Part print with two shaded views. Sizes in mm from the minimum x, y, z corner. A direction names the side the tool comes from. Coordinates: 2 decimals unless noted, no trailing zeros. Loops run counter-clockwise (first coordinate to the right, second up) from the corner with the lowest first, then second, coordinate; pieces in that order, holes last. Notation, with made-up numbers: (-11, 0) -> (15, 0) arc R26 cw to (15, 15) -> close; hole circle Ø10 at (55.5, 38). An arc over 180 degrees is marked (long way). Use one line per item in the form item = value.
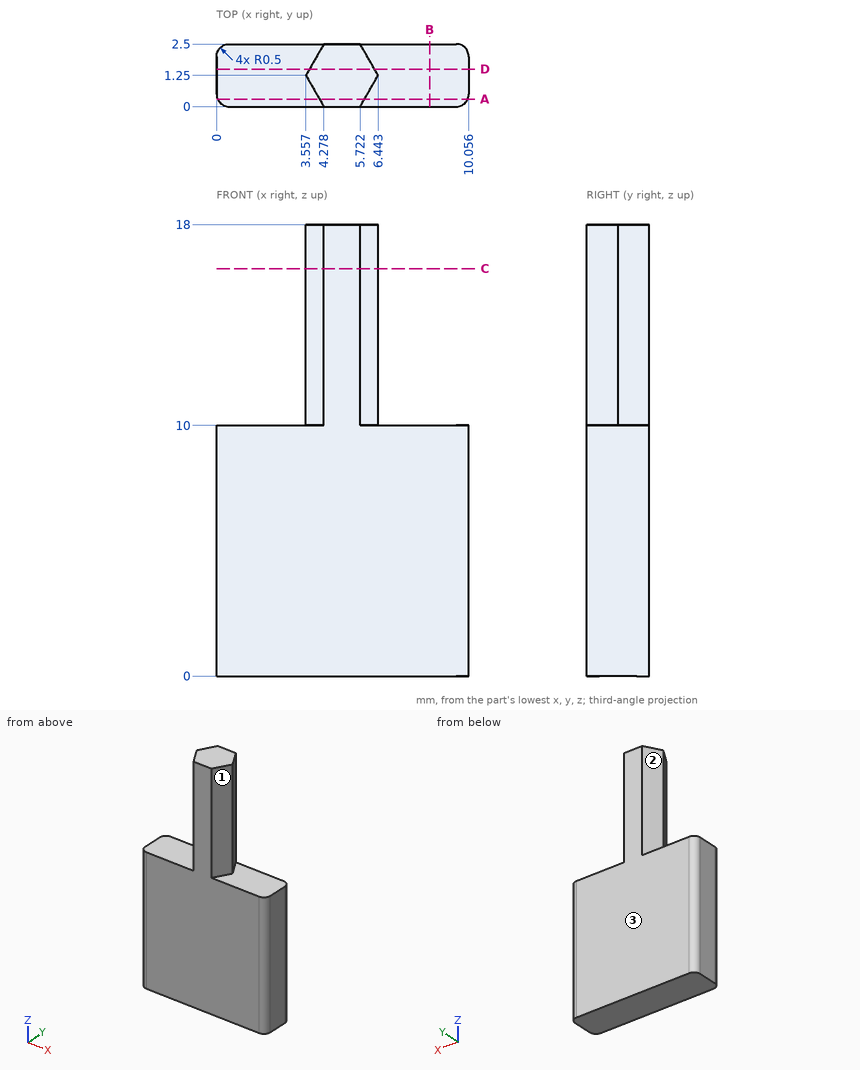
Q1. Wall check: line 1 along Z through (x, y) = (9.75, 1.5); line 2 along X through (y, z) = (0.5, 11.25); line 3 along Y through (x, z) = (6, 14) (1 decimal). Give the ranges that are in metal, low to high.
Result:
line_1 = 0 to 10
line_2 = 3.99 to 6.01
line_3 = 0.5 to 2
Q2. Which spindle directions (+Z, -Z, +X, -X, +Y, -Y) get a long thin tool onto all of the face, cutting with end or side? Do the marked faces 1, 2 and 3. Say none if no direction does.
Result:
face_1 = +Z, +X, -Y
face_2 = +Z, -X, +Y
face_3 = +Z, -Z, +X, -X, +Y
Q3. Band-saw the part on D-D, the plane y = 1.5. Write the cut outline in (x, z), and give its area (3 significant figures).
Result:
outline = (0, 0) -> (10.06, 0) -> (10.06, 10) -> (6.3, 10) -> (6.3, 18) -> (3.7, 18) -> (3.7, 10) -> (0, 10) -> close
area = 121 mm2
Q4. Band-saw the part on B-B, the plane x = 8.5. Write the cut outline in (y, z), and give its area (3 significant figures).
Result:
outline = (0, 0) -> (2.5, 0) -> (2.5, 10) -> (0, 10) -> close
area = 25.0 mm2
Q5. Band-saw the part on C-C, the plane z = 16.25. Write the cut outline in (x, y).
Result:
outline = (3.56, 1.25) -> (4.28, 0) -> (5.72, 0) -> (6.44, 1.25) -> (5.72, 2.5) -> (4.28, 2.5) -> close
Q6. Pin check, flat tips, straight feed: pin 1 Ø0.8 at (x, y) = (2, 1) entering from +Z; pin 2 Ø1.5 at (x, z) = (5.5, 7) entering from -Y. Stop position of each tip, or through.
Result:
pin_1 = 10
pin_2 = 0
Q7. Band-saw the part on A-A, the plane y = 0.3. Write the cut outline in (x, z) (1 decimal), and give its area (3 significant figures).
Result:
outline = (0, 0) -> (10, 0) -> (10, 10) -> (5.9, 10) -> (5.9, 18) -> (4.1, 18) -> (4.1, 10) -> (0, 10) -> close
area = 114 mm2
